```python
from build123d import *

# Parameters (mm, degrees)
V10_NFC_V3_REFERENCE42P7X40P4_START       = -10
SKETCH_2_W                                = 42.7
SKETCH_2_H                                = 40.4
V10_NFC_V3_REFERENCE42P7X40P4_DEPTH       = 1.6
V10_NFC_CENTRAL_COMPONENT_REFERENCE_START = -8.4
SKETCH_3_W                                = 10
SKETCH_3_H                                = 10
V10_NFC_CENTRAL_COMPONENT_REFERENCE_DEPTH = 2.2
SKETCH_5_R                                = 1.5
V12_NFC_TWO_DIAGONAL_PHOTO_HOLES_D3_DEPTH = 1.6


with BuildPart() as part:
    # 草图2 → V10_NFC_V3_reference42p7x40p4 (new body)
    with BuildSketch(Plane.XY.offset(V10_NFC_V3_REFERENCE42P7X40P4_START)):
        with Locations((100, 70)):
            Rectangle(SKETCH_2_W, SKETCH_2_H)
    extrude(amount=V10_NFC_V3_REFERENCE42P7X40P4_DEPTH)

    # 草图3 → V10_NFC_central_component_reference (add)
    with BuildSketch(Plane.XY.offset(V10_NFC_CENTRAL_COMPONENT_REFERENCE_START)):
        with Locations((100, 70)):
            Rectangle(SKETCH_3_W, SKETCH_3_H)
    extrude(amount=V10_NFC_CENTRAL_COMPONENT_REFERENCE_DEPTH)

    # 草图5 → V12_NFC_two_diagonal_photo_holes_D3 (cut)
    with BuildSketch(Plane.XY.offset(-8.4)):
        with Locations((86, 57.5)):
            Circle(SKETCH_5_R)
        with Locations((114, 82.5)):
            Circle(SKETCH_5_R)
    extrude(amount=-V12_NFC_TWO_DIAGONAL_PHOTO_HOLES_D3_DEPTH, mode=Mode.SUBTRACT)


solid = part.part
```
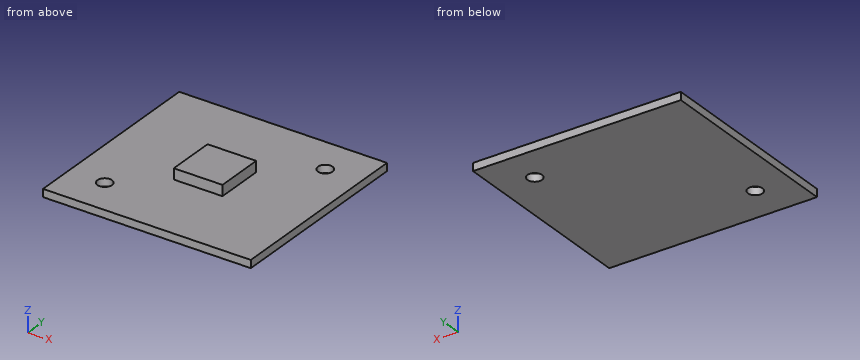
Here's how the part is built. I have some questions about the finished solid (model axes, mm). Give positions to 0.01 mm unless a question says otherwise; leave off trailing zeros. Loops run counter-clockwise (first coordinate to the right, second up) from the corner with the lowest first, then second, coordinate; pieces in that order, holes last. Notation, with made-up numbers: M 4.5,18 L 28.5,18 A20 cw 28.5,37 Z; hole C -11,55.5 d10. An arc over 180 degrees is marked long. Use one line per item in the form item = value. Start each with the question number.
Q1. Will these pins go through, and if not, where does the flat tip stop? pin 1 Ø3 at (x, y) = (95, 80.5) entering from +Z; pin 2 Ø1.1 at (y, z) = (71, -7.5) entering from +X; pin 3 Ø0.7 at (x, z) = (98.5, -7.5) entering from +Y.
Q2. If we section it at C-C (y = 68): Write out the boundary of the cut face in (x, z).
Q3. If we section it at A-A (x = 114): Write out the boundary of the cut face in (y, z).
Q4. If we section it at D-D (x = 98): Write out the boundary of the cut face in (y, z).
Q5. I need wall thicknesses on line 1 along Y through (x, z) = (114, -9.5); line 2 along X through (y, z) = (82.5, -8.9); line 3 along Z through (x, y) = (93.5, 66). Which ranges of each line are inside material? Lowest first, please.
Q6. If we section it at B-B (y = 57.5): Write out the boundary of the cut face in (x, z).
Taken from the geometry:
q1.pin_1 = -8.4
q1.pin_2 = 105
q1.pin_3 = 75
q2.outline = M 78.65,-10 L 121.35,-10 L 121.35,-8.4 L 105,-8.4 L 105,-6.2 L 95,-6.2 L 95,-8.4 L 78.65,-8.4 Z
q3.outline = M 49.8,-10 L 81,-10 L 81,-8.4 L 49.8,-8.4 Z; M 84,-10 L 90.2,-10 L 90.2,-8.4 L 84,-8.4 Z
q4.outline = M 49.8,-10 L 90.2,-10 L 90.2,-8.4 L 75,-8.4 L 75,-6.2 L 65,-6.2 L 65,-8.4 L 49.8,-8.4 Z
q5.line_1 = 49.8 to 81, 84 to 90.2
q5.line_2 = 78.65 to 112.5, 115.5 to 121.35
q5.line_3 = -10 to -8.4
q6.outline = M 78.65,-10 L 84.5,-10 L 84.5,-8.4 L 78.65,-8.4 Z; M 87.5,-10 L 121.35,-10 L 121.35,-8.4 L 87.5,-8.4 Z
